from build123d import *

# Parameters (mm, degrees)
MODEL_R             = 3.5
EXTRUDE_1_DEPTH     = 40
SKETCH_3_W          = 37
SKETCH_3_H          = 37
CUT_EXTRUDE_1_DEPTH = 40
SKETCH_4_R          = 1.5
CUT_EXTRUDE_2_DEPTH = 40


with BuildPart() as part:
    # Model → 凸台-拉伸1 (new body)
    with BuildSketch(Plane.XY):
        with BuildLine():
            Line((2619.766714505, 1592.826425633), (2619.766714505, 1613.326425633))
            Line((2619.766714505, 1613.326425633), (2592.766714505, 1613.326425633))
            Line((2592.766714505, 1613.326425633), (2592.766714505, 1592.826425633))
            ThreePointArc((2592.766714505, 1592.826425633), (2606.266714505, 1579.326425633), (2619.766714505, 1592.826425633))
        make_face()
        with Locations((2606.266714505, 1592.826425633)):
            Circle(MODEL_R, mode=Mode.SUBTRACT)
    extrude(amount=EXTRUDE_1_DEPTH)

    # 草图3 → 切除-拉伸1 (cut)
    with BuildSketch(Plane(origin=(2619.766714505, 0, 0), x_dir=(0, 0, -1), z_dir=(1, 0, 0))):
        with Locations((-21.5, 1591.826425633)):
            Rectangle(SKETCH_3_W, SKETCH_3_H)
    extrude(amount=-CUT_EXTRUDE_1_DEPTH, mode=Mode.SUBTRACT)

    # 草图4 → 切除-拉伸2 (cut)
    with BuildSketch(Plane(origin=(0, 1613.326425633, 0), x_dir=(1, 0, 0), z_dir=(0, 1, 0))):
        with Locations(Location((2600.766714505, -32, 0), (0, 0, 270))):
            Circle(SKETCH_4_R)
        with Locations(Location((2611.766714505, -32, 0), (0, 0, 270))):
            Circle(SKETCH_4_R)
        with Locations(Location((2600.766714505, -12, 0), (0, 0, 270))):
            Circle(SKETCH_4_R)
        with Locations(Location((2611.766714505, -12, 0), (0, 0, 270))):
            Circle(SKETCH_4_R)
    extrude(amount=-CUT_EXTRUDE_2_DEPTH, mode=Mode.SUBTRACT)


solid = part.part
Here's how the part is built. I have some questions about the finished solid (model axes, mm). A direction names the side the tool comes from. Round coordinates to 2 decimals unless told otherwise and drop trailing zeros. Loops run counter-clockwise (first coordinate to the right, second up) from the corner with the lowest first, then second, coordinate; pieces in that order, holes last.
1. Which directions (+Z, -Z, +X, -X, +Y, -Y) give clear straight access to the entire face, cutting with the end or side of a thin tool? Please do faces 4 (the face through (2606, 1610.326, 22)), 5 (the face through (2619.767, 1611, 14)).
Answer list:
face 4: +Z, +X, -X, -Y
face 5: +Z, -Z, +X, +Y, -Y
2. We'd pull the mould along Y, two halves only. Please class faces 1 (the face through (2610.302, 1611.847, 11.675)), 2 (the face through (2606, 1613.326, 20)), 3 (the face through (2602.77, 1592.98, 1.48)): +Y half, -Y half, draft (parallel to the pull), parting line (faces both ways), or undercut.
Answer list:
face 1: draft
face 2: +Y half
face 3: undercut
3. If we section it at C-C on y = 1598: Write out the boundary of the cut face in (x, z).
Answer list:
outline: (2592.77, 0) - (2619.77, 0) - (2619.77, 3) - (2592.77, 3) - close
4. If we section it at A-A on z = 11: Write out the boundary of the cut face in (x, y), plus the area to 3 significant figures.
Answer list:
outline: (2592.77, 1610.33) - (2599.65, 1610.33) - (2599.65, 1613.33) - (2592.77, 1613.33) - close; (2601.88, 1610.33) - (2610.65, 1610.33) - (2610.65, 1613.33) - (2601.88, 1613.33) - close; (2612.88, 1610.33) - (2619.77, 1610.33) - (2619.77, 1613.33) - (2612.88, 1613.33) - close
area: 67.6 mm2
5. For P1, Ø4, axis at x = 2599, y = 1600, coming from the +Z side; P2, Ø2.5, axis at x = 2600.77, z = 12, coming from the +Y side, each with a flat end and sliding along its axis, tell me the tip position at first contact or that it passes through.
Answer list:
P1: stops at z = 3
P2: passes through
6. If I drill on line 1 along X through (y, z) = (1611.2, 12); line 2 along Y through (x, z) = (2595.5, 18); line 3 along Z through (x, y) = (2612.25, 1581), over which ranges is the centre line in solid material (lowest first)?
Answer list:
line 1: x = 2592.77 to 2599.27, 2602.27 to 2610.27, 2613.27 to 2619.77
line 2: y = 1610.33 to 1613.33
line 3: z = 0 to 3
7. If we section it at D-D on z = 26.5: Write out the boundary of the cut face in (x, y).
Answer list:
outline: (2592.77, 1610.33) - (2619.77, 1610.33) - (2619.77, 1613.33) - (2592.77, 1613.33) - close
8. If we section it at B-B on x = 2606.5: Write out the boundary of the cut face in (y, z), plus the area to 3 significant figures.
Answer list:
outline: (1579.33, 0) - (1589.33, 0) - (1589.33, 3) - (1579.33, 3) - close; (1596.32, 0) - (1613.33, 0) - (1613.33, 40) - (1610.33, 40) - (1610.33, 3) - (1596.32, 3) - close
area: 192 mm2
